```python
from build123d import *

# Parameters (mm, degrees)
SKETCH_1_W          = 444
SKETCH_1_H          = 1106
EXTRUDE_305_DEPTH   = 116
CUT_EXTRUDE_1_DEPTH = 70


with BuildPart() as part:
    # Эскиз1 → Extrude 305 (new body)
    with BuildSketch(Plane(origin=(0, 0, 0), x_dir=(1, 0, 0), z_dir=(0, 1, 0))):
        with Locations((222, 553)):
            Rectangle(SKETCH_1_W, SKETCH_1_H)
    extrude(amount=-EXTRUDE_305_DEPTH)

    # Эскиз2 → Вырез-Вытянуть1 (cut)
    with BuildSketch(Plane(origin=(0, 0, 0), x_dir=(1, 0, 0), z_dir=(0, 1, 0))):
        Polygon((242, 1047), (202, 1047), (202, 1017), (77, 1017), (77, 904), (202, 904), (202, 854), (92, 854), (92, 741), (202, 741), (202, 691), (92, 691), (92, 578), (202, 578), (202, 528), (92, 528), (92, 415), (202, 415), (202, 365), (92, 365), (92, 252), (202, 252), (202, 202), (127, 202), (127, 89), (202, 89), (202, 59), (242, 59), (242, 89), (317, 89), (317, 202), (242, 202), (242, 252), (352, 252), (352, 365), (242, 365), (242, 415), (352, 415), (352, 528), (242, 528), (242, 578), (352, 578), (352, 691), (242, 691), (242, 741), (352, 741), (352, 854), (242, 854), (242, 904), (367, 904), (367, 1017), (242, 1017), align=None)
    extrude(amount=-CUT_EXTRUDE_1_DEPTH, mode=Mode.SUBTRACT)


solid = part.part
```
CAD build for the part. Positions are in the model's coordinates, mm. A direction names the side the tool comes from. Round coordinates to 2 decimals unless told otherwise and drop trailing zeros. Order: outer loops, then holes, each group sorted by start corner. A loop starts at its lowest first (then second) coordinate and runs counter-clockwise, first axis right, second up. Notation, with made-up numbers: (83.5, -16) -> (113.5, -16) arc R21 ccw to (113.5, 19) -> close; hole circle Ø10 at (9.25, 69.25). An arc over 180 degrees is marked (long way). One line per question, with ' | ' between items.
Q1. Drop a flat-ended pin along its axis: pin 1 (10 mm diameter, centred on x = 151.5, z = -588.5, fed in from +Y). Give the stop position or say it passes through.
Completed:
pin 1: stops at y = -70
Q2. Probe probe 1 along Z at (x, y) = (101, -36); probe 2 along X at (y, z) = (-42, -195); probe 3 along X at (y, z) = (-8.5, -70). List the from-to ranges inside material, lowest first.
Completed:
probe 1: z = -1106 to -1017, -904 to -854, -741 to -691, -578 to -528, -415 to -365, -252 to 0 | probe 2: x = 0 to 127, 317 to 444 | probe 3: x = 0 to 202, 242 to 444
Q3. Slice it at A-A (x = 261). Write the cut outline in (y, z), then the cut area to 3 significant figures.
Completed:
outline: (-116, -1106) -> (0, -1106) -> (0, -1017) -> (-70, -1017) -> (-70, -904) -> (0, -904) -> (0, -854) -> (-70, -854) -> (-70, -741) -> (0, -741) -> (0, -691) -> (-70, -691) -> (-70, -578) -> (0, -578) -> (0, -528) -> (-70, -528) -> (-70, -415) -> (0, -415) -> (0, -365) -> (-70, -365) -> (-70, -252) -> (0, -252) -> (0, -202) -> (-70, -202) -> (-70, -89) -> (0, -89) -> (0, 0) -> (-116, 0) -> close | area: 80,800 mm^2
Q4. Slice it at B-B (z = -110.5). Write the cut outline in (x, y).
Completed:
outline: (0, -116) -> (444, -116) -> (444, 0) -> (317, 0) -> (317, -70) -> (127, -70) -> (127, 0) -> (0, 0) -> close
Q5. Slice it at C-C (z = -875.5). Write the cut outline in (x, y), then the cut area to 3 significant figures.
Completed:
outline: (0, -116) -> (444, -116) -> (444, 0) -> (242, 0) -> (242, -70) -> (202, -70) -> (202, 0) -> (0, 0) -> close | area: 48,700 mm^2
Q6. Which spindle directions (+Z, -Z, +X, -X, +Y, -Y) get a long thin tool onto all of the face, cutting with end or side? Do faces 1 (the flat face through (219, -57, -1106)), 2 (the flat face through (146, -35, -578)). Say none if no direction does.
Completed:
face 1: -Z, +X, -X, +Y, -Y | face 2: +Y
Q7. Two-plate mould, pull along Z, no slides. Class faces 3 (the flat face through (92, -35, -472)), 4 (the flat face through (444, -57, -545)), 5 (the flat face through (219, -57, 0)): released by +Z, released by -Z, zero draft, split by the parting line, or undercut.
Completed:
face 3: undercut | face 4: zero draft | face 5: released by +Z
